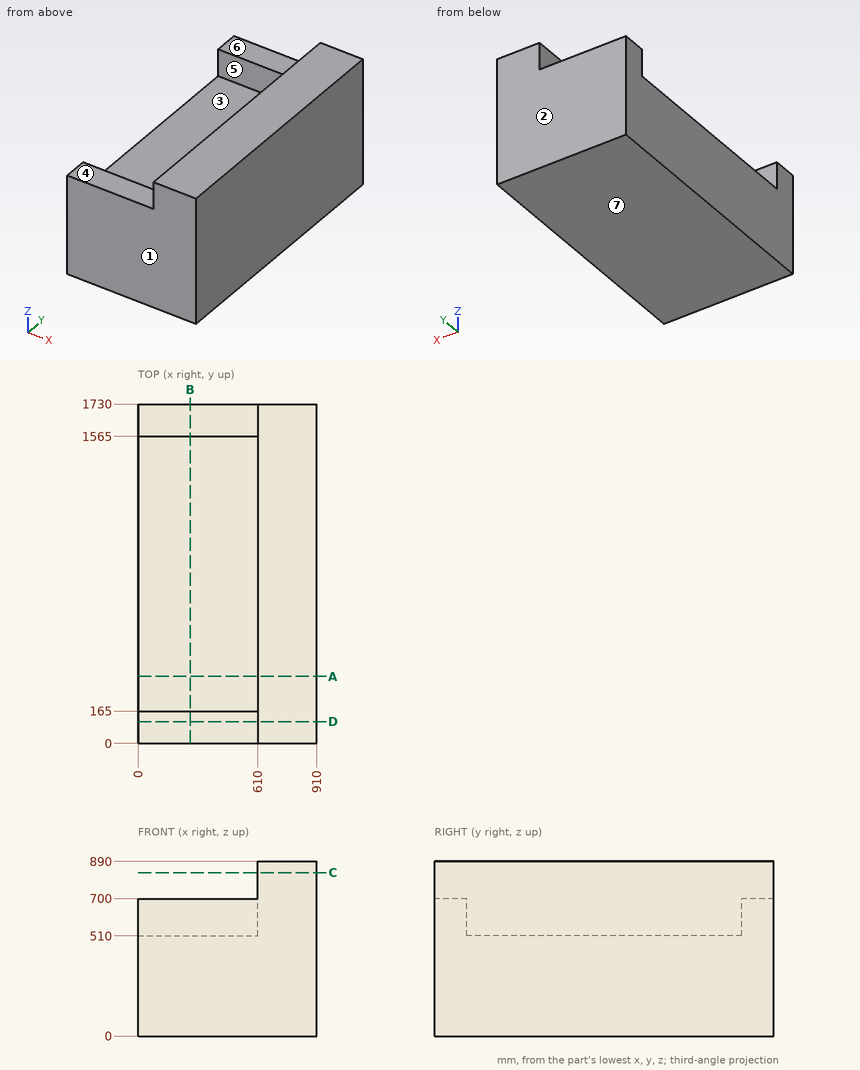
Answer from the drawing. Dimensions are ordinates in mm from the lowest x, y and z of the part. A direction names the side the tool comes from. Give positions to 0.01 mm unless a question says otherwise; leave off trailing zeros. Order: outer loops, then holes, each group sorted by start corner. A loop starts at its lowest first (then second) coordinate and runs counter-clockwise, first axis right, second up. Notation, with made-up numbers: (-16, 48.25) -> (12, 48.25) arc R18 cw to (12, 70.25) -> close; hole circle Ø3 at (68, 13.5). An arc over 180 degrees is marked (long way). Answer as a JSON object with one key per item and string values. Group by question number.
1. Section B-B on x = 266 is taken. Determine the outline of the cut face in (y, z).
2. Section A-A on y = 341 is taken. Determine the outline of the cut face in (x, z).
3. Section C-C on z = 833 is taken. Determine the outline of the cut face in (x, y).
4. The mould has two halves that part along Y. Classify the marked faces 1, 2, 3 and 4: released by +Y, released by -Y, zero draft, split by the parting line, or undercut.
5. Consider line 1 along Y through (x, z) = (144, 590); line 2 along Z through (x, y) = (501, 665); line 3 along X through (y, z) = (681.5, 589.5). Determine where each line is inside the solid, lowest interval first. Write a range as [from, to].
6. A tool of negligible diameter and unlimited length cuts with its end or side. For the marked faces 5, 6 and 7, from which of +Z, -Z, +X, -X, +Y, -Y can it reach the whole face along a straight path? Write none if from no direction.
7. Section D-D on y = 111.5 is taken. Determine the outline of the cut face in (x, z), plus the area to 3 significant figures.
Result sheet:
{
 "1": {"outline": "(0, 0) -> (1730, 0) -> (1730, 700) -> (1565, 700) -> (1565, 510) -> (165, 510) -> (165, 700) -> (0, 700) -> close"},
 "2": {"outline": "(0, 0) -> (910, 0) -> (910, 890) -> (610, 890) -> (610, 510) -> (0, 510) -> close"},
 "3": {"outline": "(610, 0) -> (910, 0) -> (910, 1730) -> (610, 1730) -> close"},
 "4": {"face 1": "released by -Y", "face 2": "released by +Y", "face 3": "undercut", "face 4": "zero draft"},
 "5": {"line 1": "y = [0, 165], [1565, 1730]", "line 2": "z = [0, 510]", "line 3": "x = [610, 910]"},
 "6": {"face 5": "+Z, -X", "face 6": "+Z, -X, +Y, -Y", "face 7": "-Z, +X, -X, +Y, -Y"},
 "7": {"outline": "(0, 0) -> (910, 0) -> (910, 890) -> (610, 890) -> (610, 700) -> (0, 700) -> close", "area": "694,000 mm^2"}
}
